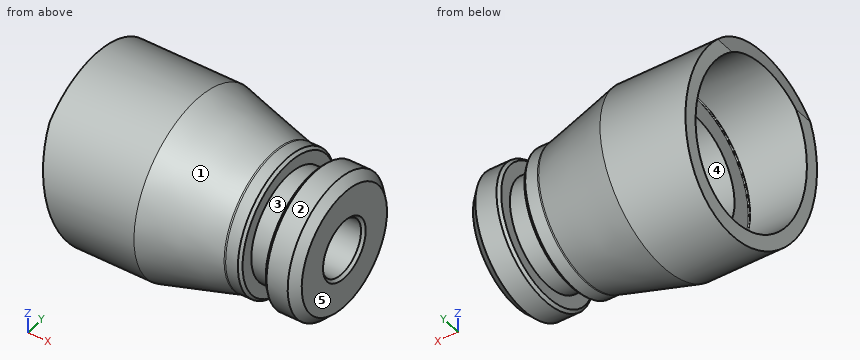
from build123d import *

# Parameters (mm, degrees)
CUT_EXTRUDE_12_DEPTH      = 102.948516419
CUT_EXTRUDE_12_DEPTH_BACK = 102.948516419


with BuildPart() as part:
    # Эскиз1 → Revolve 236 (revolve)
    with BuildSketch(Plane.XY, mode=Mode.PRIVATE) as revolve_236_sk:
        with BuildLine():
            Line((0, 32.5), (37, 32.5))
            Line((37, 32.5), (64.745695, 25.068113))
            ThreePointArc((64.745695, 25.068113), (65.002224223, 25.017098236), (65.263217049, 24.999995817))
            Line((65.263217049, 24.999995817), (69.749999449, 24.999995817))
            Line((69.749999449, 24.999995817), (70.749999449, 23.999995817))
            Line((70.749999449, 23.999995817), (70.749999449, 19.499995817))
            Line((70.749999449, 19.499995817), (79.25, 19.499995817))
            Line((79.25, 19.499995817), (79.25, 24))
            Line((79.25, 24), (80.25, 25))
            Line((80.25, 25), (88, 25))
            Line((88, 25), (91, 22))
            Line((91, 22), (91, 11))
            Line((91, 11), (90, 10))
            Line((90, 10), (61, 10))
            Line((61, 10), (61, 19))
            ThreePointArc((61, 19), (60.707106781, 19.707106781), (60, 20))
            Line((60, 20), (25, 20))
            Line((25, 20), (25, 27.1))
            ThreePointArc((25, 27.1), (24.882842712, 27.382842712), (24.6, 27.5))
            Line((24.6, 27.5), (0, 27.5))
            Line((0, 27.5), (0, 32.5))
        make_face()
    revolve(revolve_236_sk.sketch.rotate(Axis((0, 0, 0), (1, 0, 0)), 90), axis=Axis((0, 0, 0), (1, 0, 0)))

    # Эскиз2 → Наклон торца 12 градусов (cut, two sides: drawn at the far end of the back side and taken through both)
    with BuildSketch(Plane(origin=(0, 0, 0), x_dir=(1, 0, 0), z_dir=(0, 1, 0)).offset(-CUT_EXTRUDE_12_DEPTH_BACK)):
        Polygon((-25, 50), (15.30407244, 50), (-5.951583727, -50), (-25, -50), align=None)
    extrude(amount=CUT_EXTRUDE_12_DEPTH + CUT_EXTRUDE_12_DEPTH_BACK, mode=Mode.SUBTRACT)


solid = part.part
Work out the finished part from the listing and answer in its coordinate system (mm). Face numbers are marked on the shaded views. A direction names the side the tool comes from. Round coordinates to 2 decimals unless told otherwise and drop trailing zeros. Loops run counter-clockwise (first coordinate to the right, second up) from the corner with the lowest first, then second, coordinate; pieces in that order, holes last. Notation, with made-up numbers: (-37.5, -4.5) - (-3.5, -4.5) arc R13 ccw to (-3.5, 14.5) - close; hole circle Ø8 at (88.25, 32). An arc over 180 degrees is marked (long way). Use one line per item in the form item = value. Start each with the question number.
(1) Determine the mould class of the marked faces 1, 2 and 3 for opening direction X: +X half, -X half, draft (parallel to the pull), parting line (faces both ways), or undercut.
(2) Which of the six approach directions +Z, -Z, +X, -X, +Y, -Y give full straight-line access (tool end or side, diameter ignored) to the marked faces 4 and 5?
(3) Find section A-A on x = 73. Determine the outline of the cut face in (y, z), and give its area (3 significant figures).
(4) Consider line 1 (Y direction, x = 33.5, z = 0.5); line 2 (X direction, y = 20.5, z = 2.5); line 3 (Y direction, x = 5.75, z = 0). Determine where each line is inside the solid, lowest interval first.
(5) Flat-ended cylindrical pins translate along their axes: P1, Ø12, axis at y = 0, z = 0, coming from the +X side; P2, Ø5, axis at y = 24, z = -6.5, coming from the +X side; P3, Ø24, axis at y = 0, z = 0, coming from the -X side; P4, Ø6, axis at x = 60.5, z = 9.5, coming from the +Y side. Find the tip coordinate at first contact, or state that the pin passes through.
(6) Find section B-B on x = 38.5. Determine the outline of the cut face in (y, z).
Answer list:
q1.face_1 = +X half
q1.face_2 = draft
q1.face_3 = undercut
q2.face_4 = -X
q2.face_5 = +Z, -Z, +X, +Y, -Y
q3.outline = circle Ø39 at (0, 0); hole circle Ø20 at (0, 0)
q3.area = 880 mm^2
q4.line_1 = -32.5 to -19.99, 19.99 to 32.5
q4.line_2 = 25 to 70.75, 79.25 to 91
q4.line_3 = -32.5 to -27.5, 27.5 to 32.5
q5.P1 = through
q5.P2 = 90.64
q5.P3 = 61
q5.P4 = 25.74
q6.outline = circle Ø64.2 at (0, 0); hole circle Ø40 at (0, 0)
